```python
from build123d import *

# Parameters (mm, degrees)
SKETCH2_R          = 19
EXTRUDE1_DEPTH     = 3
SKETCH3_R          = 5
EXTRUDE3_DEPTH     = 1
EXTRUDE4_START     = -4
EXTRUDE4_OUTLINE_R = 3
EXTRUDE4_DEPTH     = 4
FILLET1_R          = 0.5
SCALE1_SCALE       = 0.5


# Read off the part's stored shape, not the designer's step: Extrude4
with BuildPart() as part:
    # Sketch2 → Extrude1 (new body)
    with BuildSketch(Plane.XY):
        Circle(SKETCH2_R)
    extrude(amount=EXTRUDE1_DEPTH)

    # Sketch3 → Extrude3 (add)
    with BuildSketch(Plane.XY.offset(3)):
        Circle(SKETCH3_R)
    extrude(amount=EXTRUDE3_DEPTH)

    # Extrude4 outline → Extrude4 (cut)
    with BuildSketch(Plane.XY.offset(4).offset(EXTRUDE4_START)):
        Circle(EXTRUDE4_OUTLINE_R)
    extrude(amount=EXTRUDE4_DEPTH, mode=Mode.SUBTRACT)

    # Fillet1
    fillet1_edges = [part.edges().sort_by_distance(p)[0] for p in [
        (-5, 0, 4),
    ]]
    fillet(fillet1_edges, radius=FILLET1_R)


with BuildPart() as part_1:
    # Scale1: scaled about (0, 0, 0)
    add(part.part.scale(SCALE1_SCALE))


solid = part_1.part
```
Here's how the part is built. I have some questions about the finished solid (model axes, mm). A direction names the side the tool comes from. Round coordinates to 2 decimals unless told otherwise and drop trailing zeros. Order: outer loops, then holes, each group sorted by start corner. A loop starts at its lowest first (then second) coordinate and runs counter-clockwise, first axis right, second up. Notation, with made-up numbers: (-20.5, -32) -> (33.5, -32) arc R24 ccw to (33.5, -2) -> close; hole circle Ø4 at (55.25, 82). An arc over 180 degrees is marked (long way). Use a Markdown table: item, result. Add a question column.
(1) For faces 4 (the face through (2, -2, 1.5)), 5 (the face through (-2, 0, 2)), which set-ups out of +Z, -Z, +X, -X, +Y, -Y let a thin tool reach every point of the face, with its end or its side?
(2) For pin 1 Ø1 at (y, z) = (4.5, 1.5) entering from +X; pin 2 Ø1 at (x, y) = (-1.5, -3.5) entering from +Z; pin 3 Ø2.5 at (x, y) = (0, 0) entering from +Z, each with a flat end and sliding along its axis, tell me the tip position at first contact or that it passes through.
(3) If we mould it in two halves opening along Y, with no side actions, what happens to faces 1 (the face through (4.38, -8.43, 0.74)), 2 (the face through (0, -2, 0)), 3 (the face through (-1.5, 0.07, 0.99))? For each: released by +Y, released by -Y, zero draft, split by the parting line, or undercut.
(4) Suppose I cut it at C-C, the plane z = 0.7. Please give me the cut outline in (x, y).
(5) I need wall thicknesses on line 1 along Y through (x, z) = (0, 1.25); line 2 along Z through (x, y) = (-3.25, -6.5); line 3 along X through (y, z) = (0.5, 0.35). Which ranges of each line are inside material? Lowest first, please.
(6) Suppose I cut it at A-A, the plane x = 0. Please give me the cut outline in (y, z).
(7) Suppose I cut it at D-D, the plane y = 6. Please give me the cut outline in (x, z).
Verdict:
| question | item | result |
|---|---|---|
| 1 | face 4 | +Z |
| 1 | face 5 | +Z, +X, -X, +Y, -Y |
| 2 | pin 1 | x = 8.62 |
| 2 | pin 2 | z = 1.5 |
| 2 | pin 3 | through |
| 3 | face 1 | split by the parting line |
| 3 | face 2 | zero draft |
| 3 | face 3 | undercut |
| 4 | outline | circle Ø19 at (0, 0); hole circle Ø3 at (0, 0) |
| 5 | line 1 | -9.5 to -1.5, 1.5 to 9.5 |
| 5 | line 2 | 0 to 1.5 |
| 5 | line 3 | -9.49 to -1.41, 1.41 to 9.49 |
| 6 | outline | (-9.5, 0) -> (-1.5, 0) -> (-1.5, 2) -> (-2.25, 2) arc R0.25 ccw to (-2.5, 1.75) -> (-2.5, 1.5) -> (-9.5, 1.5) -> close; (1.5, 0) -> (9.5, 0) -> (9.5, 1.5) -> (2.5, 1.5) -> (2.5, 1.75) arc R0.25 ccw to (2.25, 2) -> (1.5, 2) -> close |
| 7 | outline | (-7.37, 0) -> (7.37, 0) -> (7.37, 1.5) -> (-7.37, 1.5) -> close |
